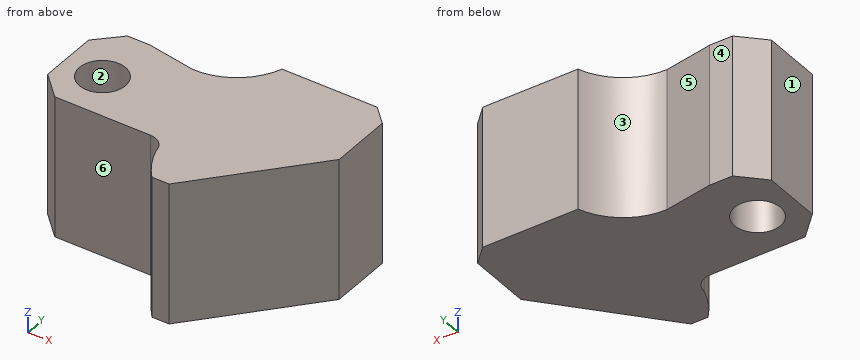
from build123d import *

# Parameters (mm, degrees)
BOSS_EXTRU_1_DEPTH      = 43
ESQUISSE2_R             = 7
ENL_V_MAT_EXTRU_1_DEPTH = 43


with BuildPart() as part:
    # Esquisse1 → Boss.-Extru.1 (new body)
    with BuildSketch(Plane.XY):
        with BuildLine():
            Line((71.055498862, 42.585779817), (100.055498862, 42.585779817))
            Line((100.055498862, 42.585779817), (105.055498862, 37.585779817))
            Line((105.055498862, 37.585779817), (105.055498862, 18.585779817))
            Line((105.055498862, 18.585779817), (76.055498862, -14.414220183))
            Line((76.055498862, -14.414220183), (70.843566259, -14.414220183))
            ThreePointArc((70.843566259, -14.414220183), (67.503369178, -9.678966252), (65.171321088, -4.374147872))
            ThreePointArc((65.171321088, -4.374147872), (63.610652231, -1.028725087), (60.179844427, 0.334029003))
            Line((60.179844427, 0.334029003), (31.055498862, 0.334029003))
            Line((31.055498862, 0.334029003), (24.055498862, 7.334029003))
            Line((24.055498862, 7.334029003), (24.055498862, 25.334029003))
            Line((24.055498862, 25.334029003), (31.055498862, 32.334029003))
            Line((31.055498862, 32.334029003), (38.055498862, 32.334029003))
            Line((38.055498862, 32.334029003), (52.765077496, 29.740333415))
            ThreePointArc((52.765077496, 29.740333415), (63.998851376, 33.189185585), (71.055498862, 42.585779817))
        make_face()
    extrude(amount=BOSS_EXTRU_1_DEPTH)

    # Esquisse2 → Enlèv. mat.-Extru.1 (cut)
    with BuildSketch(Plane.XY.offset(43)):
        with Locations((35.888461386, 14.334029003)):
            Circle(ESQUISSE2_R)
    extrude(amount=-ENL_V_MAT_EXTRU_1_DEPTH, mode=Mode.SUBTRACT)


solid = part.part
Check sheet for the modelled part. Datum: model origin and axes. Units: mm. Face numbers are marked on the shaded views. A direction names the side the tool comes from. Round coordinates to 2 decimals unless told otherwise and drop trailing zeros. Loops run counter-clockwise (first coordinate to the right, second up) from the corner with the lowest first, then second, coordinate; pieces in that order, holes last. Notation, with made-up numbers: (-18.5, 44.5) -> (22.5, 44.5) arc R32 cw to (22.5, 82.5) -> close; hole circle Ø9 at (37.5, 2.25). An arc over 180 degrees is marked (long way). Put each result on its own line as item: value. Start each with the question number.
1. Draft check along Y on the marked faces 1, 2 and 3. Enter one of: +Y half, -Y half, draft (parallel to the pull), parting line (faces both ways), or undercut.
2. Section check A-A (y = 20). Enter the section's corners in (x, z).
3. Access from +Z, -Z, +X, -X, +Y, -Y to the whole of each face (thin tool, end or side, straight path). Record for the marked faces 4, 5 and 6.
4. Scan lines: probe 1 along X at (y, z) = (8.5, 15); probe 2 along Y at (x, z) = (95, 23.5); probe 3 along X at (y, z) = (36, 3). Record each from-to range of solid material in increasing order.
5. Gauge pin test, flat ends, axial feed: pin 1 (7.5 mm diameter, centred on x = 33.5, z = 19.5, fed in from +Y); pin 2 (4 mm diameter, centred on x = 60, z = 33.5, fed in from -Y); pin 3 (2 mm diameter, centred on y = 35, z = 11.5, fed in from -X). Record the tip position at first contact, or that the pin passes through.
6. Section check B-B (z = 19). Enter the section's corners in (x, y), plus the area to 3 significant figures.
7. Section check D-D (y = -11). Enter the section's corners in (x, z).
8. Section check C-C (x = 79). Enter the section's corners in (y, z), plus the area to 3 significant figures.
Findings:
1. face 1: draft
1. face 2: undercut
1. face 3: +Y half
2. outline: (24.06, 0) -> (31.78, 0) -> (31.78, 43) -> (24.06, 43) -> close; (40, 0) -> (105.06, 0) -> (105.06, 43) -> (40, 43) -> close
3. face 4: +Z, -Z, -X, +Y
3. face 5: +Z, -Z, +Y
3. face 6: +Z, -Z, -X, -Y
4. probe 1: x = 24.06 to 32.02, 39.76 to 96.19
4. probe 2: y = 7.14 to 42.59
4. probe 3: x = 67.18 to 105.06
5. pin 1: stops at y = 32.33
5. pin 2: stops at y = -0.01
5. pin 3: stops at x = 65.07
6. outline: (24.06, 7.33) -> (31.06, 0.33) -> (60.18, 0.33) arc R5 cw to (65.17, -4.37) arc R29 ccw to (70.84, -14.41) -> (76.06, -14.41) -> (105.06, 18.59) -> (105.06, 37.59) -> (100.06, 42.59) -> (71.06, 42.59) arc R19 cw to (52.77, 29.74) -> (38.06, 32.33) -> (31.06, 32.33) -> (24.06, 25.33) -> close; hole circle Ø14 at (35.89, 14.33)
6. area: 2,810 mm^2
7. outline: (68.3, 0) -> (79.06, 0) -> (79.06, 43) -> (68.3, 43) -> close
8. outline: (-11.06, 0) -> (42.59, 0) -> (42.59, 43) -> (-11.06, 43) -> close
8. area: 2,310 mm^2
